Build history of the part. All positions in model axes, mm. A direction names the side the tool comes from. Coordinates: 2 decimals unless noted, no trailing zeros. Order: outer loops, then holes, each group sorted by start corner. A loop starts at its lowest first (then second) coordinate and runs counter-clockwise, first axis right, second up. Notation, with made-up numbers: (55, -30) - (108, -30) arc R27 cw to (108, -9) - close; hole circle Ø4 at (-20.75, 13.5). An arc over 180 degrees is marked (long way). Write each question's results on one line, items separated by ' | '.
from build123d import *

# Parameters (mm, degrees)
F1_DEPTH = 200


with BuildPart() as f1:
    # F0 (on Front) → F1 (new body)
    with BuildSketch(Plane.XZ):
        with BuildLine():
            Line((32.5, 69.5), (32.5, 80))
            Line((32.5, 80), (-32.5, 80))
            Line((-32.5, 80), (-32.5, -80))
            Line((-32.5, -80), (32.5, -80))
            Line((32.5, -80), (32.5, -69.5))
            Line((32.5, -69.5), (-19, -69.5))
            ThreePointArc((-19, -69.5), (-23.242641, -67.742641), (-25, -63.5))
            Line((-25, -63.5), (-25, 63.5))
            ThreePointArc((-25, 63.5), (-23.242641, 67.742641), (-19, 69.5))
            Line((-19, 69.5), (32.5, 69.5))
        make_face()
    extrude(amount=-F1_DEPTH)


solid = f1.part
1. Tool access for faces 1 (the face through (32.5, 99, 75)), 2 (the face through (6, 99, 69.5)): list every direction of +Z, -Z, +X, -X, +Y, -Y with a clear straight run to the whole face (end or side of a thin tool).
Solved:
face 1: +Z, -Z, +X, +Y, -Y | face 2: +X, +Y, -Y
2. Two-plate mould, pull along Z, no slides. Class faces 3 (the face through (7, 99, -69.5)), 4 (the face through (0, 99, 80)), 5 (the face through (0, 99, -80)), 6 (the face through (-32.5, 99, 1)): +Z half, -Z half, draft (parallel to the pull), parting line (faces both ways), or undercut.
Solved:
face 3: undercut | face 4: +Z half | face 5: -Z half | face 6: draft
3. Band-saw the part on C-C on z = 32. Give the cut face in (x, y).
Solved:
outline: (-32.5, 0) - (-25, 0) - (-25, 200) - (-32.5, 200) - close
4. Band-saw the part on A-A on x = -13. Give the cut face in (y, z), then the cut area to 3 significant figures.
Solved:
outline: (0, -80) - (200, -80) - (200, -69.5) - (0, -69.5) - close; (0, 69.5) - (200, 69.5) - (200, 80) - (0, 80) - close | area: 4,200 mm2
5. Probe line 1 (Z direction, x = -10, y = 136); line 2 (X direction, y = 191, z = -62); line 3 (Z direction, x = -20.5, y = 186). List the from-to ranges inside material, lowest first.
Solved:
line 1: z = -80 to -69.5, 69.5 to 80 | line 2: x = -32.5 to -25 | line 3: z = -80 to -69.31, 69.31 to 80
6. Band-saw the part on B-B on y = 128. Give the cut face in (x, z).
Solved:
outline: (-32.5, -80) - (32.5, -80) - (32.5, -69.5) - (-19, -69.5) arc R6 cw to (-25, -63.5) - (-25, 63.5) arc R6 cw to (-19, 69.5) - (32.5, 69.5) - (32.5, 80) - (-32.5, 80) - close
7. Drop flat-ended pins along their axis: pin 1 Ø12 at (y, z) = (67.5, 60) entering from +X; pin 2 Ø3 at (y, z) = (123, -24.5) entering from +X. Give the stop position or say it passes through.
Solved:
pin 1: stops at x = -24.45 | pin 2: stops at x = -25
